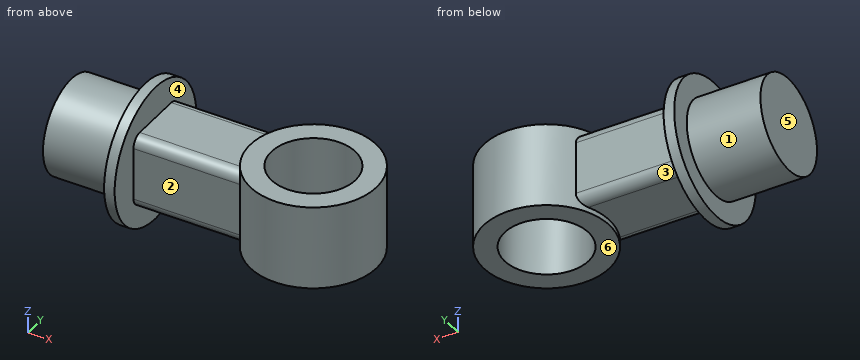
```python
from build123d import *

# Parameters (mm, degrees)
SKETCH1_R           = 45
BOSS_EXTRUDE1_DEPTH = 70
SKETCH2_R           = 65
BOSS_EXTRUDE2_DEPTH = 10
SKETCH3_R           = 60
SKETCH3_R_2         = 40
BOSS_EXTRUDE3_DEPTH = 40
SKETCH4_W           = 70
SKETCH4_H           = 70
BOSS_EXTRUDE4_DEPTH = 110
FILLET1_R           = 10


with BuildPart() as part:
    # Sketch1 → Boss-Extrude1 (new body)
    with BuildSketch(Plane(origin=(0, 0, 0), x_dir=(0, 0, -1), z_dir=(1, 0, 0))):
        Circle(SKETCH1_R)
    extrude(amount=BOSS_EXTRUDE1_DEPTH)

    # Sketch2 → Boss-Extrude2 (add)
    with BuildSketch(Plane(origin=(70, 0, 0), x_dir=(0, 0, -1), z_dir=(1, 0, 0))):
        Circle(SKETCH2_R)
    extrude(amount=BOSS_EXTRUDE2_DEPTH)



with BuildPart() as body_2:
    # Sketch3 → Boss-Extrude3 (new, symmetric)
    with BuildSketch(Plane.XY):
        with Locations((230, 0)):
            Circle(SKETCH3_R)
        with Locations((230, 0)):
            Circle(SKETCH3_R_2, mode=Mode.SUBTRACT)
    extrude(amount=BOSS_EXTRUDE3_DEPTH, both=True)


with BuildPart() as part_1:
    add(part.part)

    add(body_2.part)  # Boss-Extrude4 merges body 2
    # Sketch4 → Boss-Extrude4 (add)
    with BuildSketch(Plane(origin=(80, 0, 0), x_dir=(0, 0, -1), z_dir=(1, 0, 0))):
        Rectangle(SKETCH4_W, SKETCH4_H)
    extrude(amount=BOSS_EXTRUDE4_DEPTH)

    # Fillet1
    fillet1_edges = [part_1.edges().sort_by_distance(p)[0] for p in [
        (130.633014138, -35, -35),
        (130.633014138, -35, 35),
        (130.633014138, 35, 35),
        (130.633014138, 35, -35),
    ]]
    fillet(fillet1_edges, radius=FILLET1_R)


solid = part_1.part
```
Design review of the part built by this model. Coordinates are the model's own, in mm. Face numbers are marked on the shaded views. A direction names the side the tool comes from. Give positions to 0.01 mm unless a question says otherwise; leave off trailing zeros. Write each loop counter-clockwise with the first axis right and the second up, starting at its lowest first coordinate (ties: lowest second). Pieces come first, ordered by that corner, then holes. Notation, with made-up numbers: (85.25, -32) -> (116.25, -32) arc R17 ccw to (116.25, -24) -> close; hole circle Ø10 at (35.5, 20.5). An arc over 180 degrees is marked (long way). Answer in a Markdown table with one row per item.
(1) Consider section B-B (x = 230). State the section outline as (y, z) points, then the cut area to 3 significant figures.
Results:
| item | result |
|---|---|
| outline | (-60, -40) -> (-40, -40) -> (-40, 40) -> (-60, 40) -> close; (40, -40) -> (60, -40) -> (60, 40) -> (40, 40) -> close |
| area | 3,200 mm2 |
(2) To check wall thickness, follow probe 1 along X at (y, z) = (0, 19.5); probe 2 along Y at (x, z) = (230, 12); probe 3 along X at (y, z) = (-36, -31). State the ranges of each line that lie inside material, in increasing order.
Results:
| item | result |
|---|---|
| probe 1 | 0 to 190, 270 to 290 |
| probe 2 | -60 to -40, 40 to 60 |
| probe 3 | 70 to 80, 182 to 212.56, 247.44 to 278 |
(3) Consider section C-C (y = 0). State the section outline as (x, z) points.
Results:
| item | result |
|---|---|
| outline | (0, -45) -> (70, -45) -> (70, -65) -> (80, -65) -> (80, -35) -> (170, -35) -> (170, -40) -> (190, -40) -> (190, 40) -> (170, 40) -> (170, 35) -> (80, 35) -> (80, 65) -> (70, 65) -> (70, 45) -> (0, 45) -> close; (270, -40) -> (290, -40) -> (290, 40) -> (270, 40) -> close |
(4) Consider section A-A (z = 0). State the section outline as (x, y) points, then the cut area to 3 significant figures.
Results:
| item | result |
|---|---|
| outline | (0, -45) -> (70, -45) -> (70, -65) -> (80, -65) -> (80, -35) -> (181.27, -35) arc R60 ccw (long way) to (181.27, 35) -> (80, 35) -> (80, 65) -> (70, 65) -> (70, 45) -> (0, 45) -> close; hole circle Ø80 at (230, 0) |
| area | 20,400 mm2 |
(5) Clearance check with flat-ended pins moving along their axes: pin 1 (1 mm diameter, centred on x = 87.5, y = -28.5, fed in from -Z); pin 2 (5 mm diameter, centred on x = 179.5, y = -36.5, fed in from -Z); pin 3 (10 mm diameter, centred on x = 88, z = -13, fed in from +Y). State where each tip first meets the part, or that it passes through.
Results:
| item | result |
|---|---|
| pin 1 | z = -34.54 |
| pin 2 | z = -40 |
| pin 3 | y = 35 |
(6) Consider section D-D (z = 15). State the section outline as (x, y) points.
Results:
| item | result |
|---|---|
| outline | (0, -42.43) -> (70, -42.43) -> (70, -63.25) -> (80, -63.25) -> (80, -35) -> (181.27, -35) arc R60 ccw (long way) to (181.27, 35) -> (80, 35) -> (80, 63.25) -> (70, 63.25) -> (70, 42.43) -> (0, 42.43) -> close; hole circle Ø80 at (230, 0) |
(7) Mouldability with a two-part tool opening along X and no side actions: class the marked faces 4, 5 and 6 as +X half, -X half, draft (parallel to the pull), parting line (faces both ways), or undercut.
Results:
| item | result |
|---|---|
| face 4 | undercut |
| face 5 | -X half |
| face 6 | draft |
(8) For the marked faces 1, 2 and 3, list the 3-axis set-ups (+Z, -Z, +X, -X, +Y, -Y) from which the entire face can be reached by the end or side of a thin tool; tool diameter is ignored.
Results:
| item | result |
|---|---|
| face 1 | -X |
| face 2 | +Z, -Z, -Y |
| face 3 | -Z, +Y |
